from build123d import *

# Parameters (mm, degrees)
SKETCH002_R  = 7
PAD_DEPTH    = 22
SKETCH001_R  = 30
PAD001_DEPTH = 2
SKETCH_R     = 3
PAD002_DEPTH = 7
PAD003_DEPTH = 101
PAD004_DEPTH = 35
SKETCH007_R  = 3
SKETCH007_W  = 5
SKETCH007_H  = 5
POCKET_DEPTH = 15
CHAMFER_SIZE = 0.5


with BuildPart() as part:
    # Sketch002 → Pad (new body)
    with BuildSketch(Plane.XY):
        Circle(SKETCH002_R)
    extrude(amount=PAD_DEPTH)

    # Sketch001 → Pad001 (new body)
    with BuildSketch(Plane(origin=(0, 0, 0), x_dir=(1, 0, 0), z_dir=(0, 0, -1))):
        Circle(SKETCH001_R)
    extrude(amount=PAD001_DEPTH)

    # Sketch → Pad002 (new body)
    with BuildSketch(Plane(origin=(0, 0, -2), x_dir=(1, 0, 0), z_dir=(0, 0, -1))):
        with BuildLine():
            ThreePointArc((-34.800013, 42.799987), (-40.456858, 40.456845), (-42.8, 34.800001))
            Line((-42.8, 34.800001), (-42.8, -34.800026))
            ThreePointArc((-42.8, -34.800026), (-40.456849, -40.456854), (-34.800013, -42.799987))
            Line((-34.800013, -42.799987), (34.800013, -42.799987))
            ThreePointArc((34.800013, -42.799987), (40.456853, -40.45685), (42.8, -34.800013))
            Line((42.8, 34.800013), (42.8, -34.800013))
            ThreePointArc((42.8, 34.800013), (40.456853, 40.45685), (34.800013, 42.799987))
            Line((-34.800013, 42.799987), (34.800013, 42.799987))
        make_face()
        with Locations((-34.800013, 34.8)):
            Circle(SKETCH_R, mode=Mode.SUBTRACT)
        with Locations((34.800013, 34.8)):
            Circle(SKETCH_R, mode=Mode.SUBTRACT)
        with Locations((34.800013, -34.8)):
            Circle(SKETCH_R, mode=Mode.SUBTRACT)
        with Locations((-34.800013, -34.8)):
            Circle(SKETCH_R, mode=Mode.SUBTRACT)
    extrude(amount=PAD002_DEPTH)

    # Sketch003 → Pad003 (new body)
    with BuildSketch(Plane(origin=(0, 0, -9), x_dir=(1, 0, 0), z_dir=(0, 0, -1))):
        with BuildLine():
            ThreePointArc((-34.799995, 26.8), (-29.143142, 29.143149), (-26.8, 34.800005))
            Line((-26.8, 34.800005), (-26.8, 42.8))
            Line((-26.8, 42.8), (26.8, 42.8))
            Line((26.8, 42.8), (26.8, 34.800007))
            ThreePointArc((26.8, 34.800007), (29.143141, 29.14315), (34.799995, 26.8))
            Line((34.799995, 26.8), (42.8, 26.8))
            Line((42.8, 26.8), (42.8, -26.8))
            Line((42.8, -26.8), (34.799993, -26.8))
            ThreePointArc((34.799993, -26.8), (29.143141, -29.143151), (26.8, -34.800007))
            Line((26.8, -42.8), (26.8, -34.800007))
            Line((-26.8, -42.8), (26.8, -42.8))
            Line((-26.8, -34.800007), (-26.8, -42.8))
            ThreePointArc((-26.8, -34.800007), (-29.143141, -29.143151), (-34.799993, -26.8))
            Line((-42.8, -26.8), (-34.799993, -26.8))
            Line((-42.8, 26.8), (-42.8, -26.8))
            Line((-34.799995, 26.8), (-42.8, 26.8))
        make_face()
    extrude(amount=PAD003_DEPTH)

    # Sketch006 → Pad004 (new body)
    with BuildSketch(Plane(origin=(0, 0, -110), x_dir=(1, 0, 0), z_dir=(0, 0, -1))):
        with BuildLine():
            ThreePointArc((15, 20), (14.220252, 23.537936), (10.725728, 22.582266))
            Line((10.725728, 22.582266), (9.539937, 20.377429))
            ThreePointArc((9.539937, 20.377429), (-2.71517, 22.335574), (-14.144211, 17.498322))
            Line((-15.823725, 19.354837), (-14.144211, 17.498322))
            ThreePointArc((-15.823725, 19.354837), (-19.445436, 19.445436), (-19.354837, 15.823725))
            Line((-19.354837, 15.823725), (-17.498325, 14.144208))
            ThreePointArc((-17.498325, 14.144208), (-22.5, -1e-05), (-17.498313, -14.144223))
            Line((-17.498313, -14.144223), (-19.354837, -15.823725))
            ThreePointArc((-19.354837, -15.823725), (-19.445436, -19.445436), (-15.823725, -19.354837))
            Line((-14.144223, -17.498313), (-15.823725, -19.354837))
            ThreePointArc((-14.144223, -17.498313), (-2.715178, -22.335573), (9.539937, -20.377429))
            Line((9.539937, -20.377429), (10.725728, -22.582266))
            ThreePointArc((10.725728, -22.582266), (14.220252, -23.537936), (15, -20))
            Line((42.8, -20), (15, -20))
            Line((42.8, 20), (42.8, -20))
            Line((15, 20), (42.8, 20))
        make_face()
    extrude(amount=PAD004_DEPTH)

    # Sketch007 → Pocket (cut)
    with BuildSketch(Plane.XY.offset(22)):
        Circle(SKETCH007_R)
        with Locations((0, 7)):
            Rectangle(SKETCH007_W, SKETCH007_H)
    extrude(amount=-POCKET_DEPTH, mode=Mode.SUBTRACT)

    # Chamfer
    chamfer_edges = [part.edges().sort_by_distance(p)[0] for p in [
        (-3.968627, -5.766281, 22),
    ]]
    chamfer(chamfer_edges, length=CHAMFER_SIZE)


solid = part.part
Read the model definition and answer for the solid it produces. Units are mm, in the model's axes. A direction names the side the tool comes from. Give positions to 0.01 mm unless a question says otherwise; leave off trailing zeros. Write each loop counter-clockwise with the first axis right and the second up, starting at its lowest first coordinate (ties: lowest second). Pieces come first, ordered by that corner, then holes. Notation, with made-up numbers: (-12.5, 53) - (1.5, 53) arc R18 ccw to (1.5, 75) - close; hole circle Ø1 at (-25.5, 62). An arc over 180 degrees is marked (long way). Use CSV: the item, a comma, the result in double quotes. Start each with the question number.
Item 1: The part is cut by section C-C, the plane y = -12. Give the vertices of the cut face in (x, z), and give its area (3 significant figures).
Item 2: Flat-ended cylindrical pins translate along their axes: P1, Ø2.5, axis at y = -40, z = -78.5, coming from the -X side; P2, Ø2.5, axis at x = -40, z = -53.5, coming from the -Y side; P3, Ø6, axis at x = 33, z = -21.5, coming from the +Y side. Find the tip coordinate at first contact, or state that the pin passes through.
Item 3: For faces 1 (the flat face through (-35, 38, -9)), 2 (the cylindrical face through (29.206, 29.081, -58.793)), 3 (the flat face through (-39, -26.8, -59)), determine the directions among +Z, -Z, +X, -X, +Y, -Y from which every point of the face is accessible in a straight line to the end or side of a thin tool.
Item 4: The part is cut by section A-A, the plane z = -133. Give the vertices of the cut face in (x, y).
Item 5: The part is cut by section D-D, the plane z = -91. Give the vertices of the cut face in (x, y), and give its area (3 significant figures).
Item 6: Consider line 1 (X direction, y = 34, z = -7); line 2 (X direction, y = 37, z = -47); line 3 (Z direction, x = -5, y = -26.5). Determine where each line is inside the solid, lowest interval first.
Taken from the geometry:
1,outline,"(-42.8, -110) - (-19.03, -110) - (-19.03, -145) - (42.8, -145) - (42.8, -2) - (27.5, -2) - (27.5, 0) - (-27.5, 0) - (-27.5, -2) - (-42.8, -2) - close"
1,area,"11,500 mm2"
2,P1,"x = -26.8"
2,P2,"y = -26.8"
2,P3,"y = 28.4"
3,face 1,"-Z, -X, +Y"
3,face 2,"-Z, +X, +Y"
3,face 3,"-Z, -X, -Y"
4,outline,"(-19.35, -15.82) arc R2.5 ccw (long way) to (-15.82, -19.35) - (-14.14, -17.5) arc R22.5 ccw to (9.54, -20.38) - (10.73, -22.58) arc R2.5 ccw (long way) to (15, -20) - (42.8, -20) - (42.8, 20) - (15, 20) arc R2.5 ccw (long way) to (10.73, 22.58) - (9.54, 20.38) arc R22.5 ccw to (-14.14, 17.5) - (-15.82, 19.35) arc R2.5 ccw (long way) to (-19.35, 15.82) - (-17.5, 14.14) arc R22.5 ccw to (-17.5, -14.14) - close"
5,outline,"(-42.8, -26.8) - (-34.8, -26.8) arc R8 cw to (-26.8, -34.8) - (-26.8, -42.8) - (26.8, -42.8) - (26.8, -34.8) arc R8 cw to (34.8, -26.8) - (42.8, -26.8) - (42.8, 26.8) - (34.8, 26.8) arc R8 cw to (26.8, 34.8) - (26.8, 42.8) - (-26.8, 42.8) - (-26.8, 34.8) arc R8 cw to (-34.8, 26.8) - (-42.8, 26.8) - close"
5,area,"6,360 mm2"
6,line 1,"-42.8 to -37.69, -31.91 to 31.91, 37.69 to 42.8"
6,line 2,"-26.8 to 26.8"
6,line 3,"-110 to 0"
